from build123d import *

# Parameters (mm, degrees)
SKETCH1_W               = 44
SKETCH1_H               = 32
BOSS_EXTRUDE1_DEPTH     = 11
SKETCH2_W               = 24.5
SKETCH2_H               = 15.5
CUT_EXTRUDE1_DEPTH      = 7.75
FILLET1_R               = 7.75
CUT_EXTRUDE2_DEPTH      = 40.370833113
CUT_EXTRUDE2_DEPTH_BACK = 40.370833113
SKETCH4_R               = 2.75
SKETCH4_W               = 20
SKETCH4_H               = 10.5
CUT_EXTRUDE3_DEPTH      = 30.342801502
FILLET4_R               = 5.5
SKETCH7_W               = 10
SKETCH7_H               = 10
SKETCH7_R               = 2
BOSS_EXTRUDE5_DEPTH     = 6
FILLET5_R               = 5
CUT_EXTRUDE7_START      = -3
SKETCH9_R               = 3
SKETCH9_R_2             = 2
CUT_EXTRUDE7_DEPTH      = 3
FILLET7_R               = 10.5
FILLET8_R               = 11


# Some blends are built 0.0001 mm under size
with BuildPart() as part:
    # Sketch1 → Boss-Extrude1 (new body)
    with BuildSketch(Plane(origin=(0, 0, 0), x_dir=(0, 0, -1), z_dir=(1, 0, 0))):
        Rectangle(SKETCH1_W, SKETCH1_H)
    extrude(amount=BOSS_EXTRUDE1_DEPTH)

    # Sketch2 → Cut-Extrude1 (cut)
    with BuildSketch(Plane(origin=(0, 0, 0), x_dir=(0, 0, -1), z_dir=(1, 0, 0))):
        with Locations((0, -5.25)):
            Rectangle(SKETCH2_W, SKETCH2_H)
    extrude(amount=CUT_EXTRUDE1_DEPTH, mode=Mode.SUBTRACT)

    # Fillet1
    fillet1_edges = [part.edges().sort_by_distance(p)[0] for p in [
        (7.75, 2.5, 0),
        (7.75, -13, 0),
    ]]
    fillet(fillet1_edges, radius=FILLET1_R - 0.0001)  # a hair under: the kernel refuses the full size

    # Sketch3 → Cut-Extrude2 (cut, two sides: drawn at the far end of the back side and taken through both)
    with BuildSketch(Plane.XY.offset(-12.25).offset(-CUT_EXTRUDE2_DEPTH_BACK)):
        with BuildLine():
            ThreePointArc((0, -10.25), (3.535533906, -8.785533906), (5, -5.25))
            ThreePointArc((5, -5.25), (3.535533906, -1.714466094), (0, -0.25))
            Line((0, -0.25), (0, -10.25))
        make_face()
        with BuildLine():
            Line((0, -10.25), (0, -0.25))
            ThreePointArc((0, -0.25), (-5, -5.25), (0, -10.25))
        make_face()
    extrude(amount=CUT_EXTRUDE2_DEPTH + CUT_EXTRUDE2_DEPTH_BACK, mode=Mode.SUBTRACT)

    # Sketch4 → Cut-Extrude3 (cut, through all)
    with BuildSketch(Plane(origin=(11, 0, 0), x_dir=(0, 0, -1), z_dir=(1, 0, 0))):
        with Locations((-16, 10)):
            Circle(SKETCH4_R)
        with Locations((16, 10)):
            Circle(SKETCH4_R)
        with Locations((0, 10.75)):
            Rectangle(SKETCH4_W, SKETCH4_H)
    extrude(amount=-CUT_EXTRUDE3_DEPTH, mode=Mode.SUBTRACT)

    # Fillet4
    fillet4_edges = [part.edges().sort_by_distance(p)[0] for p in [
        (5.5, 16, 22),
        (5.5, 16, -22),
    ]]
    fillet(fillet4_edges, radius=FILLET4_R)

    # Sketch7 → Boss-Extrude5 (add)
    with BuildSketch(Plane(origin=(0, 0, 0), x_dir=(0, 0, -1), z_dir=(1, 0, 0))):
        with Locations((0, -21)):
            Rectangle(SKETCH7_W, SKETCH7_H)
        with Locations((0, -21)):
            Circle(SKETCH7_R, mode=Mode.SUBTRACT)
    extrude(amount=BOSS_EXTRUDE5_DEPTH)

    # Fillet5
    fillet5_edges = [part.edges().sort_by_distance(p)[0] for p in [
        (3, -26, -5),
        (3, -26, 5),
    ]]
    fillet(fillet5_edges, radius=FILLET5_R - 0.0001)  # a hair under: the kernel refuses the full size

    # Sketch9 → Cut-Extrude7 (cut)
    with BuildSketch(Plane(origin=(6, 0, 0), x_dir=(0, 0, -1), z_dir=(1, 0, 0)).offset(CUT_EXTRUDE7_START)):
        with Locations((0, -21)):
            Circle(SKETCH9_R)
        with Locations((0, -21)):
            Circle(SKETCH9_R_2, mode=Mode.SUBTRACT)
    extrude(amount=CUT_EXTRUDE7_DEPTH, mode=Mode.SUBTRACT)

    # Fillet7
    fillet7_edges = [part.edges().sort_by_distance(p)[0] for p in [
        (11, 5.5, 0),
    ]]
    fillet(fillet7_edges, radius=FILLET7_R)

    # Fillet8
    # the kernel refuses this fillet: 11 mm, written as the material it takes off along each edge
    with BuildSketch(Plane(origin=(11, -16, 49.5), x_dir=(0, 1, 0), z_dir=(0, 0, -1))) as fillet8_piece_1_section:
        with BuildLine():
            CenterArc((FILLET8_R, -FILLET8_R), FILLET8_R, 90, 90)
            Line((0, -FILLET8_R), (0, 0))
            Line((0, 0), (FILLET8_R, 0))
        make_face()
    fillet8_piece_1 = extrude(amount=99, mode=Mode.PRIVATE)
    fillet8_piece_1 = split(fillet8_piece_1, bisect_by=Plane(origin=(6, -13.119412113, 27.25), z_dir=(1, 0, 0)), keep=Keep.TOP, mode=Mode.PRIVATE)
    fillet8_piece_1 = split(fillet8_piece_1, bisect_by=Plane(origin=(9.313036117, -13.119412113, 5), z_dir=(0, 0, 1)), keep=Keep.TOP, mode=Mode.PRIVATE)
    add(fillet8_piece_1, mode=Mode.SUBTRACT)
    with BuildSketch(Plane(origin=(11, -16, 49.5), x_dir=(0, 1, 0), z_dir=(0, 0, -1))) as fillet8_piece_2_section:
        with BuildLine():
            CenterArc((FILLET8_R, -FILLET8_R), FILLET8_R, 90, 90)
            Line((0, -FILLET8_R), (0, 0))
            Line((0, 0), (FILLET8_R, 0))
        make_face()
    fillet8_piece_2 = extrude(amount=99, mode=Mode.PRIVATE)
    fillet8_piece_2 = split(fillet8_piece_2, bisect_by=Plane(origin=(6, -15.650616863, 27.25), z_dir=(-1, 0, 0)), keep=Keep.TOP, mode=Mode.PRIVATE)
    fillet8_piece_2 = split(fillet8_piece_2, bisect_by=Plane(origin=(4.102097244, -15.650616863, 5), z_dir=(0, 0, 1)), keep=Keep.TOP, mode=Mode.PRIVATE)
    add(fillet8_piece_2, mode=Mode.SUBTRACT)
    with BuildSketch(Plane(origin=(11, -16, 49.5), x_dir=(0, 1, 0), z_dir=(0, 0, -1))) as fillet8_piece_3_section:
        with BuildLine():
            CenterArc((FILLET8_R, -FILLET8_R), FILLET8_R, 90, 90)
            Line((0, -FILLET8_R), (0, 0))
            Line((0, 0), (FILLET8_R, 0))
        make_face()
    fillet8_piece_3 = extrude(amount=99, mode=Mode.PRIVATE)
    fillet8_piece_3 = split(fillet8_piece_3, bisect_by=Plane(origin=(6, -13.119412113, 0), z_dir=(1, 0, 0)), keep=Keep.TOP, mode=Mode.PRIVATE)
    fillet8_piece_3 = split(fillet8_piece_3, bisect_by=Plane(origin=(9.313036117, -13.119412113, -5), z_dir=(0, 0, 1)), keep=Keep.TOP, mode=Mode.PRIVATE)
    fillet8_piece_3 = split(fillet8_piece_3, bisect_by=Plane(origin=(9.313036117, -13.119412113, 5), z_dir=(0, 0, -1)), keep=Keep.TOP, mode=Mode.PRIVATE)
    add(fillet8_piece_3, mode=Mode.SUBTRACT)
    with BuildSketch(Plane(origin=(11, -16, 49.5), x_dir=(0, 1, 0), z_dir=(0, 0, -1))) as fillet8_piece_4_section:
        with BuildLine():
            CenterArc((FILLET8_R, -FILLET8_R), FILLET8_R, 90, 90)
            Line((0, -FILLET8_R), (0, 0))
            Line((0, 0), (FILLET8_R, 0))
        make_face()
    fillet8_piece_4 = extrude(amount=99, mode=Mode.PRIVATE)
    fillet8_piece_4 = split(fillet8_piece_4, bisect_by=Plane(origin=(6, -13.119412113, -27.25), z_dir=(1, 0, 0)), keep=Keep.TOP, mode=Mode.PRIVATE)
    fillet8_piece_4 = split(fillet8_piece_4, bisect_by=Plane(origin=(9.313036117, -13.119412113, -5), z_dir=(0, 0, -1)), keep=Keep.TOP, mode=Mode.PRIVATE)
    add(fillet8_piece_4, mode=Mode.SUBTRACT)
    with BuildSketch(Plane(origin=(11, -16, 49.5), x_dir=(0, 1, 0), z_dir=(0, 0, -1))) as fillet8_piece_5_section:
        with BuildLine():
            CenterArc((FILLET8_R, -FILLET8_R), FILLET8_R, 90, 90)
            Line((0, -FILLET8_R), (0, 0))
            Line((0, 0), (FILLET8_R, 0))
        make_face()
    fillet8_piece_5 = extrude(amount=99, mode=Mode.PRIVATE)
    fillet8_piece_5 = split(fillet8_piece_5, bisect_by=Plane(origin=(6, -15.650616863, -27.25), z_dir=(-1, 0, 0)), keep=Keep.TOP, mode=Mode.PRIVATE)
    fillet8_piece_5 = split(fillet8_piece_5, bisect_by=Plane(origin=(4.102097244, -15.650616863, -5), z_dir=(0, 0, -1)), keep=Keep.TOP, mode=Mode.PRIVATE)
    add(fillet8_piece_5, mode=Mode.SUBTRACT)


solid = part.part
The model under review builds one solid part; all positions refer to its coordinate system, in mm. A direction names the side the tool comes from. Round coordinates to 2 decimals unless told otherwise and drop trailing zeros. Loops run counter-clockwise (first coordinate to the right, second up) from the corner with the lowest first, then second, coordinate; pieces in that order, holes last. Notation, with made-up numbers: M 12,61.5 L 26,61.5 A15 ccw 26,67.5 Z; hole C -8,-28.75 d4. An arc over 180 degrees is marked long. Answer as CSV lines item,"result".
1. Draft analysis for pull direction Z (two halves, no side actions). For faces 1 (the face through (6, -5, 12.25)), 2 (the face through (5.58, 14.35, -20.43)), 3 (the face through (11, 6, -16)), state which applies: pulls with the +Z half, pulls with the -Z half, needs draft (parallel to the pull), parting line crosses it, or undercut.
Outcome:
face 1,"undercut"
face 2,"pulls with the -Z half"
face 3,"needs draft"
2. We need section B-B (y = 10). Give the boundary of the cut face in (x, z).
Outcome:
outline,"M 0,-22 L 11,-22 L 11,-18.75 L 0,-18.75 Z; M 0,-13.25 L 11,-13.25 L 11,-10 L 0,-10 Z; M 0,10 L 11,10 L 11,13.25 L 0,13.25 Z; M 0,18.75 L 11,18.75 L 11,22 L 0,22 Z"
3. For faces 4 (the face through (6, -17.6, -0.1)), 5 (the face through (3, -23, -1)), 6 (the face through (7, 10, -10)), list the 3-axis set-ups (+Z, -Z, +X, -X, +Y, -Y) from which the entire face can be reached by the end or side of a thin tool; tool diameter is ignored.
Outcome:
face 4,"+Z, -Z, +X, -Y"
face 5,"+X"
face 6,"+X, +Y"
4. To check wall thickness, follow L1, parallel to Z at x = 6.5, y = -7; L2, parallel to Y at x = 4.75, z = -1.5; L3, parallel to Y at x = 1.5, z = -14. State the ranges of each line that lie inside material, in increasing order. Write a range as [from, to].
Outcome:
L1,"z = [-22, -12.25], [12.25, 22]"
L2,"y = [-25.77, -23.6], [-18.4, -11.37], [0.87, 4.6]"
L3,"y = [-15.9, -10.02], [-0.48, 8.11], [11.89, 16]"
5. We need section D-D (x = 6.5). Give the boundary of the cut face in (y, z), plus the area to 3 significant figures.
Outcome:
outline,"M -13.87,-22 L 10.5,-22 A5.5 ccw 16,-16.5 L 16,-10 L 3.62,-10 L 3.62,10 L 16,10 L 16,16.5 A5.5 ccw 10.5,22 L -13.87,22 Z; hole M -9.47,-12.25 L -1.03,-12.25 L -1.03,12.25 L -9.47,12.25 Z; hole C 10,-16 d5.5; hole C 10,16 d5.5"
area,"799 mm2"
6. We need section A-A (z = 16). Give the boundary of the cut face in (x, y).
Outcome:
outline,"M 0,-16 A11 ccw 11,-5 L 11,7.25 L 0,7.25 L 0,-0.25 A5 cw 0,-10.25 Z; M 0,12.75 L 11,12.75 L 11,16 L 0,16 Z"
7. Insertion check: pin 1 Ø9.5 at (y, z) = (-21, 0) entering from +X; pin 2 Ø3 at (x, y) = (4, -19.5) entering from +Z; pin 3 Ø1 at (x, z) = (7, 12.5) entering from -Y. Each pin has a flat end and moves straight along its axis. Give the tip position at first contact, or say it passes through.
Outcome:
pin 1,"stops at x = 6"
pin 2,"stops at z = 5"
pin 3,"stops at y = -13.87"
